```python
from build123d import *

# Parameters (mm, degrees)
EXTRUDE_1_DEPTH = 820
SKETCH_3_W      = 10
SKETCH_3_H      = 10
EXTRUDE_2_DEPTH = 10


with BuildPart() as part:
    # Эскиз1 → Бобышка-Вытянуть1 (new body)
    with BuildSketch(Plane.XY):
        Polygon((0, 0), (0, 100), (20, 100), (20, 10), (10, 10), (10, 0), align=None)
    extrude(amount=EXTRUDE_1_DEPTH)

    # Эскиз3 → Бобышка-Вытянуть2 (add)
    with BuildSketch(Plane(origin=(10, 0, 0), x_dir=(0, 0, -1), z_dir=(1, 0, 0))):
        with Locations((-815, 5)):
            Rectangle(SKETCH_3_W, SKETCH_3_H)
        with Locations((-5, 5)):
            Rectangle(SKETCH_3_W, SKETCH_3_H)
    extrude(amount=EXTRUDE_2_DEPTH)


solid = part.part
```
Source: CAD feature listing. Evaluate the final solid. Frame: model axes, mm. Round coordinates to 2 decimals unless told otherwise and drop trailing zeros. Loops run counter-clockwise (first coordinate to the right, second up) from the corner with the lowest first, then second, coordinate; pieces in that order, holes last.
1. Ray query, L1, parallel to Z at x = 12.25, y = 9; L2, parallel to Y at x = 17.25, z = 700. Return the intervals inside material, ascending.
2. Contact query for flat-ended pins moving along their axis: pin 1 (11 mm diameter, centred on x = 12.5, z = 231, fed in from -Y); pin 2 (3 mm diameter, centred on x = 15.5, z = 105, fed in from -Y). Output: stop coordinate, or through.
3. Section query B-B on z = 218. Output: boundary loops of the cut face in (x, y), and give its area (3 significant figures).
4. Section query A-A on x = 16. Output: boundary loops of the cut face in (y, z), and give its area (3 significant figures).
Answers below:
1. L1: z = 0 to 10, 810 to 820
1. L2: y = 10 to 100
2. pin 1: stops at y = 0
2. pin 2: stops at y = 10
3. outline: (0, 0) - (10, 0) - (10, 10) - (20, 10) - (20, 100) - (0, 100) - close
3. area: 1,900 mm2
4. outline: (0, 0) - (100, 0) - (100, 820) - (0, 820) - (0, 810) - (10, 810) - (10, 10) - (0, 10) - close
4. area: 74,000 mm2
